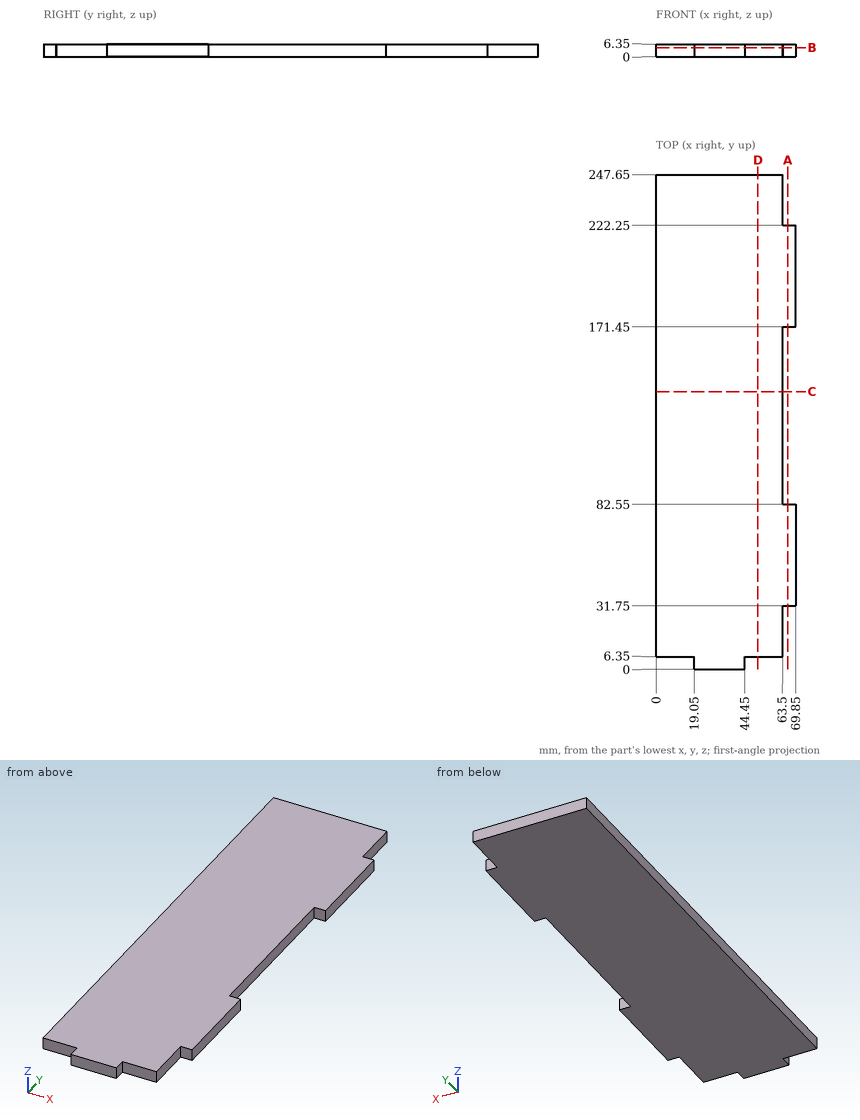
The figure shows three views and two pictorial views of one solid part (mm, origin at its lowest corner). Answer the questions. Give positions to 0.01 mm unless a question says otherwise; leave off trailing zeros. Write each loop counter-clockwise with the first axis right and the second up, starting at its lowest first coordinate (ties: lowest second). Pieces come first, ordered by that corner, then holes. Notation, with made-up numbers: M 39.25,16 L 67.25,16 A16 ccw 67.25,22 Z; hole C -31.75,-10.5 d1. An arc over 180 degrees is marked long. One line per item, written item: value. Start each with the question number.
(1) Find the intervals of material crossed by line 1 (Y direction, x = 67.5, z = 6.25); line 2 (X direction, y = 225.5, z = 3); line 3 (Y direction, x = 8, z = 5.25), in increasing order.
(2) Find section B-B (z = 4.5). Determine the outline of the cut face in (x, y), plus the area to 3 significant figures.
(3) Flat-ended cylindrical pins translate along their axes: pin 1 Ø1.9 at (x, z) = (54.5, 3.5) entering from -Y; pin 2 Ø1.9 at (y, z) = (21, 2.5) entering from +X; pin 3 Ø1.9 at (x, z) = (67.5, 3) entering from -Y. Find the tip coordinate at first contact, or state that the pin passes through.
(4) Find section C-C (y = 139). Determine the outline of the cut face in (x, z).
(5) Find section D-D (x = 51). Determine the outline of the cut face in (y, z).
(6) Find section A-A (x = 66). Determine the outline of the cut face in (y, z), plus the area to 3 significant figures.
Results below:
1. line 1: y = 31.75 to 82.55, 171.45 to 222.25
1. line 2: x = 0 to 63.5
1. line 3: y = 6.35 to 247.65
2. outline: M 0,6.35 L 19.05,6.35 L 19.05,0 L 44.45,0 L 44.45,6.35 L 63.5,6.35 L 63.5,31.75 L 69.85,31.75 L 69.85,82.55 L 63.5,82.55 L 63.5,171.45 L 69.85,171.45 L 69.85,222.25 L 63.5,222.25 L 63.5,247.65 L 0,247.65 Z
2. area: 16,100 mm^2
3. pin 1: stops at y = 6.35
3. pin 2: stops at x = 63.5
3. pin 3: stops at y = 31.75
4. outline: M 0,0 L 63.5,0 L 63.5,6.35 L 0,6.35 Z
5. outline: M 6.35,0 L 247.65,0 L 247.65,6.35 L 6.35,6.35 Z
6. outline: M 31.75,0 L 82.55,0 L 82.55,6.35 L 31.75,6.35 Z; M 171.45,0 L 222.25,0 L 222.25,6.35 L 171.45,6.35 Z
6. area: 645 mm^2
